```python
from build123d import *

# Parameters (mm, degrees)
SKETCH_1_R          = 3
EXTRUDE_1_DEPTH     = 3
SKETCH_2_R          = 1.5
CUT_EXTRUDE_1_DEPTH = 35
SKETCH_3_R          = 1.5
CUT_EXTRUDE_2_DEPTH = 10


with BuildPart() as part:
    # 草图1 → 凸台-拉伸1 (new body)
    with BuildSketch(Plane(origin=(0, 0, 0), x_dir=(1, 0, 0), z_dir=(0, 1, 0))):
        with BuildLine():
            Line((-14.251933165, 74.010414785), (-13.995374148, 76.999384294))
            Line((-13.995374148, 76.999384294), (-12.726300539, 74.013284805))
            Line((-12.726300539, 74.013284805), (-10.774799328, 76.605384534))
            ThreePointArc((-10.774799328, 76.605384534), (-10.653849778, 76.585389633), (-10.532962075, 76.565024143))
            Line((-10.532962075, 76.565024143), (-9.528973393, 73.479680611))
            Line((-9.528973393, 73.479680611), (-7.358981856, 75.891832081))
            ThreePointArc((-7.358981856, 75.891832081), (-7.240235225, 75.861371819), (-7.121582506, 75.830547768))
            Line((-7.121582506, 75.830547768), (-6.390319712, 72.669441521))
            Line((-6.390319712, 72.669441521), (-4.018352795, 74.883286801))
            ThreePointArc((-4.018352795, 74.883286801), (-3.902712818, 74.842592999), (-3.787198101, 74.801544977))
            Line((-3.787198101, 74.801544977), (-3.334226545, 71.588733941))
            Line((-3.334226545, 71.588733941), (-0.778336348, 73.587424334))
            ThreePointArc((-0.778336348, 73.587424334), (-0.666683115, 73.536806696), (-0.555185537, 73.485847103))
            Line((-0.555185537, 73.485847103), (-0.383952607, 70.245782711))
            Line((-0.383952607, 70.245782711), (2.336409001, 72.014106975))
            ThreePointArc((2.336409001, 72.014106975), (2.443225743, 71.953950731), (2.549857617, 71.893467401))
            Line((2.549857617, 71.893467401), (2.438048736, 68.650808499))
            Line((2.438048736, 68.650808499), (5.302178162, 70.175308618))
            ThreePointArc((5.302178162, 70.175308618), (5.403345471, 70.106071595), (5.504300109, 70.036524842))
            Line((5.504300109, 70.036524842), (5.110300349, 66.815950022))
            Line((5.110300349, 66.815950022), (8.096399838, 68.085023631))
            ThreePointArc((8.096399838, 68.085023631), (8.191147771, 68.007232764), (8.285656848, 67.929151881))
            Line((8.285656848, 67.929151881), (7.612464785, 64.755171662))
            Line((7.612464785, 64.755171662), (10.697808317, 65.759160344))
            ThreePointArc((10.697808317, 65.759160344), (10.785415785, 65.673407668), (10.872760029, 65.587386897))
            Line((10.872760029, 65.587386897), (9.925499062, 62.484157186))
            Line((9.925499062, 62.484157186), (13.086605309, 63.21541998))
            ThreePointArc((13.086605309, 63.21541998), (13.166405566, 63.122358125), (13.245920234, 63.029052137))
            Line((13.245920234, 63.029052137), (12.031799591, 60.020190385))
            Line((12.031799591, 60.020190385), (15.244610627, 60.473161941))
            ThreePointArc((15.244610627, 60.473161941), (15.315996344, 60.373499163), (15.387076283, 60.273618073))
            Line((15.387076283, 60.273618073), (13.915336154, 57.382023534))
            Line((13.915336154, 57.382023534), (17.155400546, 57.553256464))
            ThreePointArc((17.155400546, 57.553256464), (17.217828436, 57.447751259), (17.279932683, 57.342055221))
            Line((17.279932683, 57.342055221), (15.561773901, 54.589734677))
            Line((15.561773901, 54.589734677), (18.804432803, 54.477925795))
            ThreePointArc((18.804432803, 54.477925795), (18.857427751, 54.36738112), (18.910083656, 54.256674546))
            Line((18.910083656, 54.256674546), (16.958582445, 51.664574817))
            Line((16.958582445, 51.664574817), (20.179157265, 51.270575057))
            ThreePointArc((20.179157265, 51.270575057), (20.222315948, 51.155832223), (20.265122768, 51.040957657))
            Line((20.265122768, 51.040957657), (18.095131231, 48.628806187))
            Line((18.095131231, 48.628806187), (21.26911145, 47.955614125))
            ThreePointArc((21.26911145, 47.955614125), (21.302105404, 47.837546395), (21.334737353, 47.719378101))
            Line((21.334737353, 47.719378101), (18.962770436, 45.50553282))
            Line((18.962770436, 45.50553282), (22.066000147, 44.558271853))
            ThreePointArc((22.066000147, 44.558271853), (22.088578269, 44.437777794), (22.110786998, 44.317215104))
            Line((22.110786998, 44.317215104), (19.554896802, 42.318524712))
            Line((19.554896802, 42.318524712), (22.563758554, 41.104404068))
            ThreePointArc((22.563758554, 41.104404068), (22.57574901, 40.982400713), (22.587365497, 40.860361182))
            Line((22.587365497, 40.860361182), (19.867003889, 39.092036918))
            Line((19.867003889, 39.092036918), (22.758598428, 37.62029679))
            ThreePointArc((22.758598428, 37.62029679), (22.759909963, 37.497712656), (22.7608458, 37.375125079))
            Line((22.7608458, 37.375125079), (19.896716374, 35.85062496))
            Line((19.896716374, 35.85062496), (22.649036919, 34.132466177))
            ThreePointArc((22.649036919, 34.132466177), (22.639659553, 34.010234206), (22.629907617, 33.888031548))
            Line((22.629907617, 33.888031548), (19.643808128, 32.618957939))
            Line((19.643808128, 32.618957939), (22.235907857, 30.667456728))
            ThreePointArc((22.235907857, 30.667456728), (22.215912956, 30.546507177), (22.195547466, 30.425619474))
            Line((22.195547466, 30.425619474), (19.110203935, 29.421630793))
            Line((19.110203935, 29.421630793), (21.522355404, 27.251639255))
            ThreePointArc((21.522355404, 27.251639255), (21.491895142, 27.132892625), (21.461071091, 27.014239906))
            Line((21.461071091, 27.014239906), (18.299964844, 26.282977111))
            Line((18.299964844, 26.282977111), (20.513810124, 23.911010194))
            ThreePointArc((20.513810124, 23.911010194), (20.473116322, 23.795370217), (20.432068301, 23.6798555))
            Line((20.432068301, 23.6798555), (17.219257265, 23.226883944))
            Line((17.219257265, 23.226883944), (19.217947657, 20.670993748))
            ThreePointArc((19.217947657, 20.670993748), (19.167330019, 20.559340514), (19.116370426, 20.447842937))
            Line((19.116370426, 20.447842937), (15.876306034, 20.276610007))
            Line((15.876306034, 20.276610007), (17.644630298, 17.556248398))
            ThreePointArc((17.644630298, 17.556248398), (17.584474055, 17.449431657), (17.523990725, 17.342799782))
            Line((17.523990725, 17.342799782), (14.281331822, 17.454608664))
            Line((14.281331822, 17.454608664), (15.805831942, 14.590479238))
            ThreePointArc((15.805831942, 14.590479238), (15.736594919, 14.489311928), (15.667048166, 14.38835729))
            Line((15.667048166, 14.38835729), (12.446473346, 14.78235705))
            Line((12.446473346, 14.78235705), (13.715546954, 11.796257561))
            ThreePointArc((13.715546954, 11.796257561), (13.637756087, 11.701509628), (13.559675204, 11.607000551))
            Line((13.559675204, 11.607000551), (10.385694985, 12.280192614))
            Line((10.385694985, 12.280192614), (11.389683667, 9.194849082))
            ThreePointArc((11.389683667, 9.194849082), (11.303930991, 9.107241614), (11.217910221, 9.019897371))
            Line((11.217910221, 9.019897371), (8.114680509, 9.967158338))
            Line((8.114680509, 9.967158338), (8.845943303, 6.80605209))
            ThreePointArc((8.845943303, 6.80605209), (8.041013726, 6.131861333), (7.218665918, 5.479029897))
            ThreePointArc((7.218665918, 5.479029897), (-8.795258648, 2.184566676), (3.816136485, -8.219854535))
            ThreePointArc((3.816136485, -8.219854535), (31.986599548, 45.900244344), (-13.140159276, 86.962827432))
            Line((-13.140159276, 86.962827432), (-12.883600259, 89.951796941))
            Line((-12.883600259, 89.951796941), (-16.868945799, 90.293880168))
            Line((-16.868945799, 90.293880168), (-18.237278704, 74.352498011))
            Line((-18.237278704, 74.352498011), (-14.251933165, 74.010414785))
        make_face()
        with Locations(Location((0, 0, 0), (0, 0, 270))):
            Circle(SKETCH_1_R, mode=Mode.SUBTRACT)
    extrude(amount=EXTRUDE_1_DEPTH)

    # 草图2 → 切除-拉伸1 (cut)
    with BuildSketch(Plane(origin=(0, 3, 0), x_dir=(1, 0, 0), z_dir=(0, 1, 0))):
        with Locations(Location((-2.480429629, 5.463283706, 0), (0, 0, 270))):
            Circle(SKETCH_2_R)
        with Locations(Location((2.480429629, -5.463283706, 0), (0, 0, 270))):
            Circle(SKETCH_2_R)
    extrude(amount=-CUT_EXTRUDE_1_DEPTH, mode=Mode.SUBTRACT)

    # 草图3 → 切除-拉伸2 (cut)
    with BuildSketch(Plane(origin=(0, 3, 0), x_dir=(1, 0, 0), z_dir=(0, 1, 0))):
        with Locations(Location((27.095115734, 29.384103679, 0), (0, 0, 270))):
            Circle(SKETCH_3_R)
        with Locations(Location((22.024822818, 58.618310712, 0), (0, 0, 270))):
            Circle(SKETCH_3_R)
    extrude(amount=-CUT_EXTRUDE_2_DEPTH, mode=Mode.SUBTRACT)


solid = part.part
```
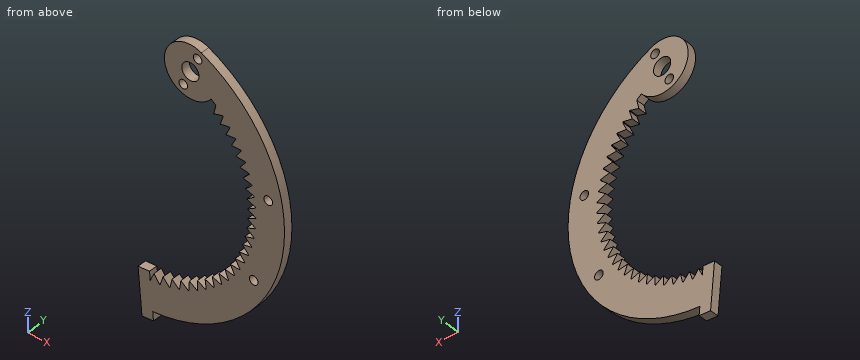
For this review, take the finished solid that the model builds, in its own axes (mm). Round coordinates to 2 decimals unless told otherwise and drop trailing zeros. Write each loop counter-clockwise with the first axis right and the second up, starting at its lowest first coordinate (ties: lowest second). Pieces come first, ordered by that corner, then holes.
1) Insertion check: pin 1 Ø1 at (y, z) = (0.5, -38.5) entering from +X; pin 2 Ø1.8 at (x, z) = (-2.48, -5.46) entering from +Y; pin 3 Ø1 at (y, z) = (1, -64.5) entering from -X. Each pin has a flat end and moves straight along its axis. Give the tip position at first contact, or say it passes through.
Answer below:
pin 1: stops at x = 32.75
pin 2: passes through
pin 3: stops at x = 7.61
2) Take a section at A-A on z = 0. Give the boundary of the cut face in (x, y).
Answer below:
outline: (-9.06, 0) - (-3, 0) - (-3, 3) - (-9.06, 3) - close; (3, 0) - (16.25, 0) - (16.25, 3) - (3, 3) - close
3) For line 1 along X through (y, z) = (0.65, -73); line 2 along X through (y, z) = (1.1, -75); line 3 along X through (y, z) = (0.55, -29), list the stretches that pass through material, from the lowest coordinate up.
Answer below:
line 1: x = -6.47 to -6.04, -3.53 to -1.53, -0.53 to 17.6
line 2: x = -18.18 to -14.17, -13.15 to -11.98, -10.02 to -8.16, -6.93 to 15.41
line 3: x = 19.58 to 25.65, 28.55 to 32.1
4) Take a section at B-B on y = 1.25. State how many separate pieces and enclosed holes the cut face has, then the cut area to 3 significant figures.
Answer below:
separate pieces: 1
enclosed holes: 5
area: 1,500 mm2
